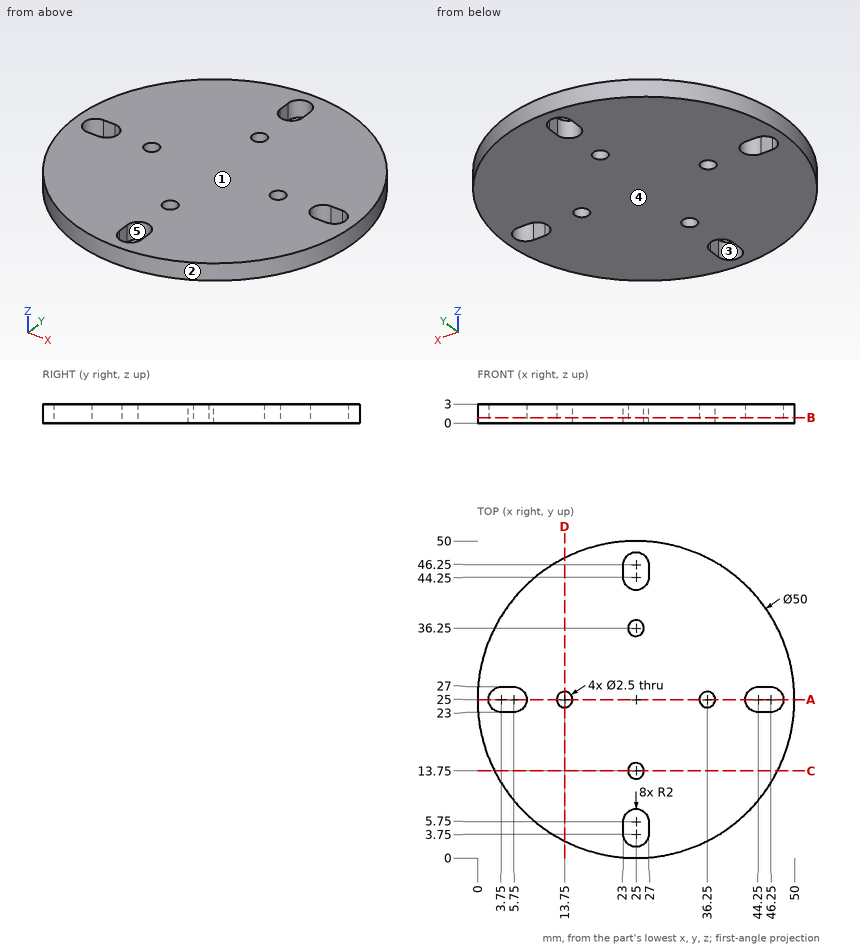
Answer from the drawing. Dimensions are ordinates in mm from the lowest x, y and z of the part. A direction names the side the tool comes from. Round coordinates to 2 decimals unless told otherwise and drop trailing zeros. Loops run counter-clockwise (first coordinate to the right, second up) from the corner with the lowest first, then second, coordinate; pieces in that order, holes last. Notation, with made-up numbers: M 26.5,40.5 L 41.5,40.5 A22 cw 41.5,61.5 Z; hole C -17.75,20.25 d10. An arc over 180 degrees is marked long. One line per question, with ' | ' between items. Start each with the question number.
(1) A tool of negligible diameter and unlimited length cuts with its end or side. For the marked faces 4 and 5, from which of +Z, -Z, +X, -X, +Y, -Y can it reach the whole face along a straight path? Write none if from no direction.
(2) A cutting plane is placed at A-A on y = 25. Write down the section's boundary in (x, z), plus the area to 3 significant figures.
(3) For a pull along X with two mould halves and no side action, classify the marked faces 1, 2 and 3 as released by +X, released by -X, zero draft, split by the parting line, or undercut.
(4) A cutting plane is placed at B-B on z = 0.85. Give the number of separate pieces and of enclosed holes in the cut face, plus the area to 3 significant figures.
(5) Find the intervals of material crossed by line 1 (Y direction, x = 25, z = 0.9); line 2 (X direction, y = 42.5, z = 0.6); line 3 (X direction, y = 36, z = 1.7), in increasing order.
(6) Flat-ended cylindrical pins translate along their axes: pin 1 Ø1.6 at (y, z) = (4.5, 2) entering from +X; pin 2 Ø1.5 at (y, z) = (9, 0.5) entering from -X; pin 3 Ø0.6 at (x, z) = (45, 1.5) entering from -Y. Find the tip coordinate at first contact, or state that the pin passes through.
(7) A cutting plane is placed at C-C on y = 13.75. Write down the section's boundary in (x, z), plus the area to 3 significant figures.
Geometry check:
1) face 4: -Z, +X, -X, +Y, -Y | face 5: +Z, -Z
2) outline: M 0,0 L 1.75,0 L 1.75,3 L 0,3 Z; M 7.75,0 L 12.5,0 L 12.5,3 L 7.75,3 Z; M 15,0 L 35,0 L 35,3 L 15,3 Z; M 37.5,0 L 42.25,0 L 42.25,3 L 37.5,3 Z; M 48.25,0 L 50,0 L 50,3 L 48.25,3 Z | area: 99.0 mm²
3) face 1: zero draft | face 2: split by the parting line | face 3: undercut
4) separate pieces: 1 | enclosed holes: 8 | area: 1,860 mm²
5) line 1: y = 0 to 1.75, 7.75 to 12.5, 15 to 35, 37.5 to 42.25, 48.25 to 50 | line 2: x = 7.15 to 24.03, 25.97 to 42.85 | line 3: x = 2.55 to 23.78, 26.22 to 47.45
6) pin 1: stops at x = 40.39 | pin 2: stops at x = 5.19 | pin 3: stops at y = 9.61
7) outline: M 2.67,0 L 23.75,0 L 23.75,3 L 2.67,3 Z; M 26.25,0 L 47.33,0 L 47.33,3 L 26.25,3 Z | area: 126 mm²
